Geometry check sheet. Reference: the model listing, model coordinates, mm. A direction names the side the tool comes from. Give positions to 0.01 mm unless a question says otherwise; leave off trailing zeros. Loops run counter-clockwise (first coordinate to the right, second up) from the corner with the lowest first, then second, coordinate; pieces in that order, holes last.
1. Cross-section at C-C, the plane y = 1.25. Record the cut outline in (x, z).
2. Cross-section at D-D, the plane z = -5. Record the cut outline in (x, y).
3. Go/stop test with flat-tipped pins: pin 1 Ø0.5 at (x, y) = (9.5, 5) entering from -Z; pin 2 Ø5 at (x, y) = (9.5, -0.5) entering from -Z; pin 3 Ø4 at (x, z) = (-1.5, -7.5) entering from -Y; pin 4 Ø6 at (x, z) = (0.5, -4) entering from -Y. Record where each tip stops, or that it passes through.
4. Cross-section at A-A, the plane x = -7.06. Record the cut outline in (y, z), plus the area to 3 significant figures.
5. Cross-section at B-B, the plane z = -1.27. Record the cut outline in (x, y), plus the area to 3 significant figures.
6. Material ranges on L1, parallel to X at y = 6.25, z = -14; L2, parallel to Z at x = 21, y = 1.25; L3, parallel to Y at x = 8, z = -9.25, recorded low to high.
7. Tool access check on faces 1 (the flat face through (-4.97, 8.6, -13.55)), 2 (the flat face through (8.3, 7.6, -11.55)). Record the directions out of +Z, -Z, +X, -X, +Y, -Y that give a thin tool (end or side, any length) a straight path to the whole face; none if there is none.
from build123d import *

# Parameters (mm, degrees)
SKETCH1_W           = 53.47
SKETCH1_H           = 12.33
BASE_EXTRUDE_DEPTH  = 12.7
BOSS_EXTRUDE1_DEPTH = 6.07
SKETCH4_R           = 0.5
CUT_EXTRUDE1_DEPTH  = 5.08
SKETCH5_R           = 0.5
CUT_EXTRUDE2_DEPTH  = 5.08
SKETCH6_R           = 0.3556
BOSS_EXTRUDE2_DEPTH = 2.54
LPATTERN1_COUNT     = 13
LPATTERN1_PITCH     = 2.7686
LPATTERN2_COUNT     = 13
LPATTERN2_PITCH     = 2.7686
LPATTERN3_COUNT     = 12
LPATTERN3_PITCH     = 2.7686
SKETCH7_R           = 0.3556
BOSS_EXTRUDE3_DEPTH = 2.54
LPATTERN4_COUNT     = 12
LPATTERN4_PITCH     = 2.7686
SKETCH12_R          = 1.304277921
BOSS_EXTRUDE4_DEPTH = 6.07
SKETCH9_W           = 6.35508
SKETCH9_H           = 10.16
CUT_EXTRUDE3_DEPTH  = 9.33
SKETCH11_R          = 1.4
CUT_EXTRUDE4_DEPTH  = 6.08
CHAMFER1_SIZE       = 0.4


with BuildPart() as part:
    # Sketch1 → Base-Extrude (new body)
    with BuildSketch(Plane(origin=(0, 0, 0), x_dir=(1, 0, 0), z_dir=(0, 1, 0))):
        with Locations((16.575, 4.395)):
            Rectangle(SKETCH1_W, SKETCH1_H)
    extrude(amount=BASE_EXTRUDE_DEPTH)

    # Sketch2 → Boss-Extrude1 (add)
    with BuildSketch(Plane(origin=(0, 0, -10.56), x_dir=(-1, 0, 0), z_dir=(0, 0, -1))):
        with BuildLine():
            Line((-32.654431338, 2.286), (-0.495568662, 2.286))
            ThreePointArc((-0.495568662, 2.286), (1.120925043, 2.8667787), (1.998186376, 4.34352118))
            Line((1.998186376, 4.34352118), (2.538755038, 7.13752118))
            ThreePointArc((2.538755038, 7.13752118), (2.0042213, 9.236493705), (0.045, 10.16))
            Line((0.045, 10.16), (-33.195, 10.16))
            ThreePointArc((-33.195, 10.16), (-35.1542213, 9.236493705), (-35.688755038, 7.13752118))
            Line((-35.688755038, 7.13752118), (-35.148186376, 4.34352118))
            ThreePointArc((-35.148186376, 4.34352118), (-34.270925043, 2.8667787), (-32.654431338, 2.286))
        make_face()
    extrude(amount=BOSS_EXTRUDE1_DEPTH)

    # Sketch4 → Cut-Extrude1 (cut)
    with BuildSketch(Plane(origin=(0, 0, -16.63), x_dir=(-1, 0, 0), z_dir=(0, 0, -1))):
        with Locations((0, 7.62)):
            Circle(SKETCH4_R)
    cut_extrude1 = extrude(amount=-CUT_EXTRUDE1_DEPTH, mode=Mode.SUBTRACT)

    # Sketch5 → Cut-Extrude2 (cut)
    with BuildSketch(Plane(origin=(0, 0, -16.63), x_dir=(-1, 0, 0), z_dir=(0, 0, -1))):
        with Locations((-1.397, 5.08)):
            Circle(SKETCH5_R)
    cut_extrude2 = extrude(amount=-CUT_EXTRUDE2_DEPTH, mode=Mode.SUBTRACT)

    # Sketch6 → Boss-Extrude2 (add)
    with BuildSketch(Plane.XZ):
        Circle(SKETCH6_R)
    boss_extrude2 = extrude(amount=BOSS_EXTRUDE2_DEPTH)

    # LPattern1: Boss-Extrude2 ×13
    with Locations(*[(i * LPATTERN1_PITCH, 0, 0) for i in range(1, LPATTERN1_COUNT)]):
        add(boss_extrude2)

    # LPattern2: Cut-Extrude1 ×13
    with Locations(*[(i * LPATTERN2_PITCH, 0, 0) for i in range(1, LPATTERN2_COUNT)]):
        add(cut_extrude1, mode=Mode.SUBTRACT)

    # LPattern3: Cut-Extrude2 ×12
    with Locations(*[(i * LPATTERN3_PITCH, 0, 0) for i in range(1, LPATTERN3_COUNT)]):
        add(cut_extrude2, mode=Mode.SUBTRACT)

    # Sketch7 → Boss-Extrude3 (add)
    with BuildSketch(Plane.XZ):
        with Locations((1.397, -2.54)):
            Circle(SKETCH7_R)
    boss_extrude3 = extrude(amount=BOSS_EXTRUDE3_DEPTH)

    # LPattern4: Boss-Extrude3 ×12
    with Locations(*[(i * LPATTERN4_PITCH, 0, 0) for i in range(1, LPATTERN4_COUNT)]):
        add(boss_extrude3)

    # Sketch12 → Boss-Extrude4 (add)
    with BuildSketch(Plane(origin=(0, 0, -10.56), x_dir=(-1, 0, 0), z_dir=(0, 0, -1))):
        Polygon((-41.595, 9.82), (-42.98, 7.421109632), (-41.595, 5.022219263), (-38.825, 5.022219263), (-37.44, 7.421109632), (-38.825, 9.82), align=None)
        with Locations((-40.21, 7.421109632)):
            Circle(SKETCH12_R, mode=Mode.SUBTRACT)
    boss_extrude4 = extrude(amount=BOSS_EXTRUDE4_DEPTH)

    # Sketch9 → Cut-Extrude3 (cut)
    with BuildSketch(Plane.XY.offset(1.77)):
        with Locations((-6.98246, 7.62)):
            Rectangle(SKETCH9_W, SKETCH9_H)
    cut_extrude3 = extrude(amount=-CUT_EXTRUDE3_DEPTH, mode=Mode.SUBTRACT)

    # Sketch11 → Cut-Extrude4 (cut, through all)
    with BuildSketch(Plane(origin=(0, 2.54, 0), x_dir=(-1, 0, 0), z_dir=(0, 1, 0))):
        with Locations((7.06, -1.27)):
            Circle(SKETCH11_R)
    cut_extrude4 = extrude(amount=-CUT_EXTRUDE4_DEPTH, mode=Mode.SUBTRACT)

    # Mirror1: Boss-Extrude4, Cut-Extrude3, Cut-Extrude4 across plane
    add(boss_extrude4.mirror(Plane(origin=(16.575, 0, 0), x_dir=(0, 0, 1), z_dir=(1, 0, 0))))
    add(cut_extrude3.mirror(Plane(origin=(16.575, 0, 0), x_dir=(0, 0, 1), z_dir=(1, 0, 0))), mode=Mode.SUBTRACT)
    add(cut_extrude4.mirror(Plane(origin=(16.575, 0, 0), x_dir=(0, 0, 1), z_dir=(1, 0, 0))), mode=Mode.SUBTRACT)

    # Chamfer1
    chamfer1_edges = [part.edges().sort_by_distance(p)[0] for p in [
        (19.8802, 7.62, -16.63),
        (22.6488, 7.62, -16.63),
        (25.4174, 7.62, -16.63),
        (28.186, 7.62, -16.63),
        (30.9546, 7.62, -16.63),
        (33.7232, 7.62, -16.63),
        (4.6656, 5.08, -16.63),
        (7.4342, 5.08, -16.63),
        (10.2028, 5.08, -16.63),
        (12.9714, 5.08, -16.63),
        (15.74, 5.08, -16.63),
        (18.5086, 5.08, -16.63),
        (21.2772, 5.08, -16.63),
        (24.0458, 5.08, -16.63),
        (26.8144, 5.08, -16.63),
        (29.583, 5.08, -16.63),
        (32.3516, 5.08, -16.63),
        (0.5, 7.62, -16.63),
        (1.897, 5.08, -16.63),
        (3.2686, 7.62, -16.63),
        (6.0372, 7.62, -16.63),
        (8.8058, 7.62, -16.63),
        (11.5744, 7.62, -16.63),
        (14.343, 7.62, -16.63),
        (17.1116, 7.62, -16.63),
    ]]
    chamfer(chamfer1_edges, length=CHAMFER1_SIZE)


solid = part.part
Result:
1. outline: (-10.16, -10.56) - (43.31, -10.56) - (43.31, 1.77) - (-10.16, 1.77) - close; hole circle Ø2.8 at (-7.06, -1.27); hole circle Ø2.8 at (40.21, -1.27)
2. outline: (-10.16, 0) - (43.31, 0) - (43.31, 2.54) - (36.95, 2.54) - (36.95, 12.7) - (-3.8, 12.7) - (-3.8, 2.54) - (-10.16, 2.54) - close
3. pin 1: stops at z = -11.55
3. pin 2: stops at z = -10.56
3. pin 3: stops at y = 0
3. pin 4: stops at y = -2.54
4. outline: (0, -10.56) - (5.02, -10.56) - (5.02, -16.63) - (6.12, -16.63) - (6.12, -10.56) - (8.73, -10.56) - (8.73, -16.63) - (9.82, -16.63) - (9.82, -10.56) - (12.7, -10.56) - (12.7, -7.56) - (2.54, -7.56) - (2.54, -2.67) - (0, -2.67) - close; (0, 0.13) - (2.54, 0.13) - (2.54, 1.77) - (0, 1.77) - close
4. area: 68.0 mm2
5. outline: (-10.16, 0) - (-8.46, 0) - (-8.46, 2.54) - (-10.16, 2.54) - close; (-5.66, 0) - (38.81, 0) - (38.81, 2.54) - (36.95, 2.54) - (36.95, 12.7) - (-3.8, 12.7) - (-3.8, 2.54) - (-5.66, 2.54) - close; (41.61, 0) - (43.31, 0) - (43.31, 2.54) - (41.61, 2.54) - close
5. area: 536 mm2
6. L1: x = -9.15 to -7.63, -6.49 to -4.97, -2.37 to 35.52, 38.12 to 39.64, 40.78 to 42.3
6. L2: z = -10.56 to 1.77
6. L3: y = 0 to 12.7
7. face 1: -Z, +Y
7. face 2: -Z
